Verification items for the finished model (mm, model axes). Round coordinates to 2 decimals unless told otherwise and drop trailing zeros. Order: outer loops, then holes, each group sorted by start corner. A loop starts at its lowest first (then second) coordinate and runs counter-clockwise, first axis right, second up. Notation, with made-up numbers: M 68.25,-24 L 81.25,-24 A10 ccw 81.25,-16 Z; hole C 84,75.25 d1. An arc over 180 degrees is marked long. Write item = value, one per line. Start each with the question number.
Autodesk Inventor part; units mm, degrees
ref_plane "YZ Plane" through (0, 0, 0) normal (1, 0, 0) x (0, 1, 0)
ref_plane "XZ Plane" through (0, 0, 0) normal (0, 1, 0) x (-1, 0, 0)
ref_plane "XY Plane" through (0, 0, 0) normal (0, 0, 1) x (1, 0, 0)
ref_plane "Work Plane1" through (0, 0, -22.225) normal (0, 0, -1) x (-1, 0, 0)
sketch "Sketch1" plane through (0, 0, -22.225) normal (0, 0, -1) x (-1, 0, 0)
  arc A0 (88.9626, 123.799) -> (43.8693, -146.1511) centre (0.2092, -0.1167) ccw
  line L0 (104.0584, 214.2592) -> (-123.3104, 207.8545)
  line L1 (104.0584, 214.2592) -> (88.9626, 123.799)
  line L2 (27.3448, -245.173) -> (43.8693, -146.1511)
  spline S0 degree 3 poles (-707.521, 203.2816) (-551.4111, 75.786) (-311.6058, 71.5174) (-123.3104, 207.8545) knots 0 0 0 0 1 1 1 1
  spline S1 degree 3 poles (-813.9039, -23.98) (-592.8487, -45.4285) (-280.1393, -149.9031) (-98.6304, -203.95) knots 0 0 0 0 1 1 1 1
  line L3 (-98.6304, -203.95) -> (27.3448, -245.173)
  arc A1 (-707.521, 203.2816) -> (-707.521, 203.2816) centre (-797.0248, 106.6489) ccw
  arc A2 (-707.521, 203.2816) -> (-707.521, 203.2816) centre (-797.0248, 106.6489) ccw
  line L4 (-754.135, 241.3513) -> (-660.9071, 165.2118) construction
  arc A3 (-742.7917, 235.6937) -> (-668.7166, 175.1963) centre (-447.712, 521.4005) ccw construction
  line L5 (-880.3002, -17.5377) -> (-747.5076, -30.4223) construction
  arc A4 (-760.9988, -30.537) -> (-867.0828, -20.2439) centre (-910.7419, -1022.0239) ccw construction
  arc A5 (-707.521, 203.2816) -> (-807.2552, -24.6472) centre (-797.0248, 106.6609) ccw
  point P0 (-439.0779, 106.766)
  point P1 (-428.475, -105.3455)
extrude "Extrusion1" add sketch "Sketch1" against normal blind 69.85
fillet "Fillet1" radius 25.4 1 edges at (-104.0584, 214.2592, 12.7)
fillet "Fillet2" radius 50.8 1 edges at (-27.3448, -245.173, 12.7)
fillet "Fillet4" radius 76.2 1 edges at (123.3104, 207.8545, 12.7)
fillet "Fillet5" radius 12.7 2 edges at (-43.8693, -146.1511, 12.7) (-88.9626, 123.799, 12.7)
properties material "Wood (Walnut)"
1) Cross-section at B-B, the plane y = 40.5. Enter the section's corners in (x, z) (3 decimals), then the cut area to 3 significant figures.
2) Scan lines: probe 1 along Y at (x, z) = (-1, -16.5); probe 2 along Y at (x, z) = (-42, 27.5); probe 3 along Y at (x, z) = (817, 10). Record each from-to range of solid material in increasing order.
3) Gauge pin test, flat ends, axial feed: P1, Ø12, axis at y = -49, z = 38, coming from the -X side; P2, Ø5, axis at x = 711, z = 24.5, coming from the +Y side. Record the tip position at first contact, or that the pin passes through.
4) Release check for a two-part mould opening along X. For faces 1 (the cylindrical face through (-85.27, 133.33, 13.19)), 2 (the flat face through (-95.587, 163.494, 12.211)), 3 (the flat face through (64.22, -215.21, 12.21)), 4 (the cylindrical face through (149.406, 28.997, 12.211)) record: pulls with the +X half, pulls with the -X half, needs draft (parallel to the pull), parting line crosses it, or undercut.
5) Cross-section at A-A, the plane x = -5.5. Enter the section's corners in (y, z) (3 decimals).
Geometry results:
q1.outline = M 146.701,-22.225 L 910.924,-22.225 L 910.924,47.625 L 146.701,47.625 Z
q1.area = 53,400 mm^2
q2.probe_1 = -227.33 to -152.54, 152.3 to 211.36
q2.probe_2 = 146.46 to 212.51
q2.probe_3 = -23.54 to 236.84
q3.P1 = 141.99
q3.P2 = 208.49
q4.face_1 = undercut
q4.face_2 = pulls with the -X half
q4.face_3 = pulls with the +X half
q4.face_4 = undercut
q5.outline = M -225.808,-22.225 L -152.446,-22.225 L -152.446,47.625 L -225.808,47.625 Z; M 152.213,-22.225 L 211.483,-22.225 L 211.483,47.625 L 152.213,47.625 Z
